Work out the finished part from the listing and answer in its coordinate system (mm). Face numbers are marked on the shaded views. A direction names the side the tool comes from. Round coordinates to 2 decimals unless told otherwise and drop trailing zeros. Loops run counter-clockwise (first coordinate to the right, second up) from the corner with the lowest first, then second, coordinate; pieces in that order, holes last. Notation, with made-up numbers: (30.5, -34) - (35.5, -34) arc R24 ccw to (35.5, -16) - close; hole circle Ø7 at (-21.75, -27). An arc over 180 degrees is marked (long way). Return JSON: item names as keys, results as strings.
from build123d import *

# Parameters (mm, degrees)
SKETCH1_W                    = 25.4
SKETCH1_H                    = 155.575
BASE_FLANGE1_DEPTH           = 1.1938
EDGE_FLANGE1_STRIP_W         = 7.7724
EDGE_FLANGE1_STRIP_H         = 1.1938
EDGE_FLANGE1_STRIP_CUT_DEPTH = 25.4
EDGE_FLANGE1_DEPTH           = 25.4
SKETCH11_R                   = 5.159375
CUT_EXTRUDE1_DEPTH           = 162.040474985
EDGE_FLANGE2_STRIP_W         = 7.7724
EDGE_FLANGE2_STRIP_H         = 1.1938
EDGE_FLANGE2_STRIP_CUT_DEPTH = 25.4
EDGE_FLANGE2_DEPTH           = 25.4
SKETCH15_R                   = 5.159375
CUT_EXTRUDE2_DEPTH           = 162.040474985


# Sheet-metal steps are written as plain solids
with BuildPart() as part:
    # Sketch1 → Base-Flange1 (new body)
    with BuildSketch(Plane(origin=(0, 0, 0), x_dir=(0, 0, -1), z_dir=(1, 0, 0))):
        with Locations((12.7, 77.7875)):
            Rectangle(SKETCH1_W, SKETCH1_H)
    extrude(amount=-BASE_FLANGE1_DEPTH)

    # Edge-Flange1 strip (across the edge) → Edge-Flange1 strip cut (cut)
    with BuildSketch(Plane(origin=(-1.1938, 155.575, 0), x_dir=(0, -1, 0), z_dir=(0, 0, -1))):
        with Locations((-1.1938, -0.5969)):
            Rectangle(EDGE_FLANGE1_STRIP_W, EDGE_FLANGE1_STRIP_H)
    extrude(amount=EDGE_FLANGE1_STRIP_CUT_DEPTH, mode=Mode.SUBTRACT)

    # Edge-Flange1 section (across the edge) → Edge-Flange1 (add)
    with BuildSketch(Plane(origin=(-1.1938, 155.575, 0), x_dir=(0, -1, 0), z_dir=(0, 0, -1))):
        with BuildLine():
            Line((0, 1.4986), (0, 31.75))
            Line((0, 31.75), (1.1938, 31.75))
            Line((1.1938, 31.75), (1.1938, 1.4986))
            ThreePointArc((1.1938, 1.4986), (1.632729778, 0.438929778), (2.6924, 0))
            Line((2.6924, 0), (2.6924, -1.1938))
            ThreePointArc((2.6924, -1.1938), (0.788585702, -0.405214298), (0, 1.4986))
        make_face()
    extrude(amount=EDGE_FLANGE1_DEPTH)

    # Sketch11 → Cut-Extrude1 (cut, through all)
    with BuildSketch(Plane(origin=(0, 155.575, 0), x_dir=(1, 0, 0), z_dir=(0, 1, 0))):
        with Locations(Location((-21.03755, 12.7, 0), (0, 0, 180))):
            Circle(SKETCH11_R)
    extrude(amount=-CUT_EXTRUDE1_DEPTH, mode=Mode.SUBTRACT)

    # Edge-Flange2 strip (across the edge) → Edge-Flange2 strip cut (cut)
    with BuildSketch(Plane.YX):
        with Locations((-1.1938, -0.5969)):
            Rectangle(EDGE_FLANGE2_STRIP_W, EDGE_FLANGE2_STRIP_H)
    extrude(amount=EDGE_FLANGE2_STRIP_CUT_DEPTH, mode=Mode.SUBTRACT)

    # Edge-Flange2 section (across the edge) → Edge-Flange2 (add)
    with BuildSketch(Plane.YX):
        with BuildLine():
            Line((0, 1.4986), (0, 31.75))
            Line((0, 31.75), (1.1938, 31.75))
            Line((1.1938, 31.75), (1.1938, 1.4986))
            ThreePointArc((1.1938, 1.4986), (1.632729778, 0.438929778), (2.6924, 0))
            Line((2.6924, 0), (2.6924, -1.1938))
            ThreePointArc((2.6924, -1.1938), (0.788585702, -0.405214298), (0, 1.4986))
        make_face()
    extrude(amount=EDGE_FLANGE2_DEPTH)

    # Sketch15 → Cut-Extrude2 (cut, through all)
    with BuildSketch(Plane.XZ):
        with Locations((19.84375, -12.7)):
            Circle(SKETCH15_R)
    extrude(amount=-CUT_EXTRUDE2_DEPTH, mode=Mode.SUBTRACT)


solid = part.part
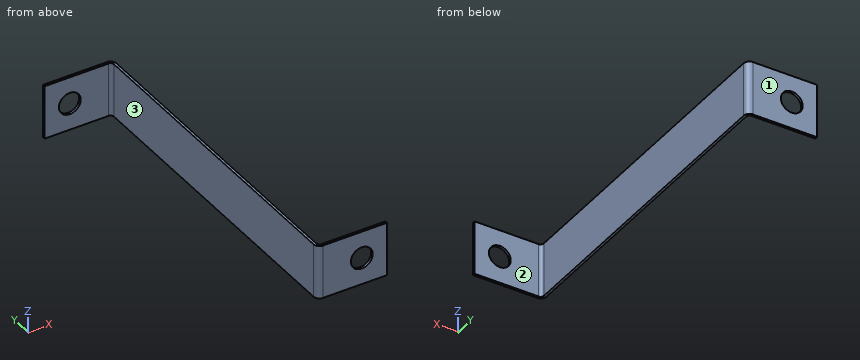
1) Find the intervals of material crossed by L1, parallel to Y at x = 8.5, z = -20; L2, parallel to Y at x = -5, z = -10.25 (3 decimals); L3, parallel to X at y = 15, z = -9.25, in increasing order.
Verdict:
{"L1": "y = 0 to 1.19", "L2": "y = 154.381 to 155.575", "L3": "x = -1.19 to 0"}
2) Section B-B (x = 21.5) is taken. Give the vertices of the cut face in (y, z).
Verdict:
{"outline": "(0, -25.4) - (1.19, -25.4) - (1.19, -17.59) - (0, -17.59) - close; (0, -7.81) - (1.19, -7.81) - (1.19, 0) - (0, 0) - close"}
3) Flat-ended cylindrical pins translate along their axes: pin 1 (5 mm diameter, centred on y = 35.5, z = -6, fed in from -X); pin 2 (12.5 mm diameter, centred on y = 114, z = -13.5, fed in from +X); pin 3 (6 mm diameter, centred on x = -21.04, z = -12.7, fed in from +Y); pin 4 (1.5 mm diameter, centred on x = -1, z = -6, fed in from -Y). Find the tip coordinate at first contact, or state that the pin passes through.
Verdict:
{"pin 1": "stops at x = -1.19", "pin 2": "stops at x = 0", "pin 3": "passes through", "pin 4": "stops at y = 0.65"}
4) Section D-D (y = 140.5) is taken. Give the vertices of the cut face in (x, z), and give its area (3 significant figures).
Verdict:
{"outline": "(-1.19, -25.4) - (0, -25.4) - (0, 0) - (-1.19, 0) - close", "area": "30.3 mm2"}
5) Section C-C (z = -5) is taken. Give the vertices of the cut face in (x, y) (3 decimals).
Verdict:
{"outline": "(-32.944, 154.381) - (-2.692, 154.381) arc R1.499 cw to (-1.194, 152.883) - (-1.194, 2.692) arc R2.692 ccw to (1.499, 0) - (31.75, 0) - (31.75, 1.194) - (1.499, 1.194) arc R1.499 cw to (0, 2.692) - (0, 152.883) arc R2.692 ccw to (-2.692, 155.575) - (-32.944, 155.575) - close"}
6) A tool of negligible diameter and unlimited length cuts with its end or side. For the marked faces 1, 2 and 3, from which of +Z, -Z, +X, -X, +Y, -Y can it reach the whole face along a straight path? Write none if from no direction.
Verdict:
{"face 1": "+Z, -Z, +X, -X, +Y", "face 2": "+Z, -Z, +X, +Y", "face 3": "+Z, -Z, -X, -Y"}
7) Section A-A (z = -12.7) is taken. Give the vertices of the cut face in (x, y) (3 decimals).
Verdict:
{"outline": "(-32.944, 154.381) - (-26.197, 154.381) - (-26.197, 155.575) - (-32.944, 155.575) - close; (-15.878, 154.381) - (-2.692, 154.381) arc R1.499 cw to (-1.194, 152.883) - (-1.194, 2.692) arc R2.692 ccw to (1.499, 0) - (14.684, 0) - (14.684, 1.194) - (1.499, 1.194) arc R1.499 cw to (0, 2.692) - (0, 152.883) arc R2.692 ccw to (-2.692, 155.575) - (-15.878, 155.575) - close; (25.003, 0) - (31.75, 0) - (31.75, 1.194) - (25.003, 1.194) - close"}
